Source: CAD feature listing. Evaluate the final solid. Frame: model axes, mm. Face numbers are marked on the shaded views. Coordinates: 2 decimals unless noted, no trailing zeros. Order: outer loops, then holes, each group sorted by start corner. A loop starts at its lowest first (then second) coordinate and runs counter-clockwise, first axis right, second up.
```python
from build123d import *

# Parameters (mm, degrees)
SKETCH1_W                = 9.525
SKETCH1_H                = 5.8
BOSS_EXTRUDE1_DEPTH      = 5.8
M3_CLEARANCE_HOLE1_D     = 3.2
M3_CLEARANCE_HOLE1_DEPTH = 12.7
M3_CLEARANCE_HOLE1_TIP   = 0.96137699
SKETCH5_R                = 0.5
CUT_EXTRUDE1_DEPTH       = 5.8


with BuildPart() as part:
    # Sketch1 → Boss-Extrude1 (new body)
    with BuildSketch(Plane.XY):
        with Locations((4.7625, 2.9)):
            Rectangle(SKETCH1_W, SKETCH1_H)
    extrude(amount=BOSS_EXTRUDE1_DEPTH)

    # M3 Clearance Hole1
    with Locations(Plane.XY.offset(5.8)):
        with Locations((6.35, 2.9)):
            Hole(M3_CLEARANCE_HOLE1_D / 2, depth=M3_CLEARANCE_HOLE1_DEPTH)
            with Locations((0, 0, -(M3_CLEARANCE_HOLE1_DEPTH + M3_CLEARANCE_HOLE1_TIP / 2))):  # 118° drill point
                Cone(0, M3_CLEARANCE_HOLE1_D / 2, M3_CLEARANCE_HOLE1_TIP, mode=Mode.SUBTRACT)

    # Sketch5 → Cut-Extrude1 (cut)
    with BuildSketch(Plane.XY.offset(5.8)):
        with Locations((2.38125, 4.2125)):
            Circle(SKETCH5_R)
    extrude(amount=-CUT_EXTRUDE1_DEPTH, mode=Mode.SUBTRACT)


solid = part.part
```
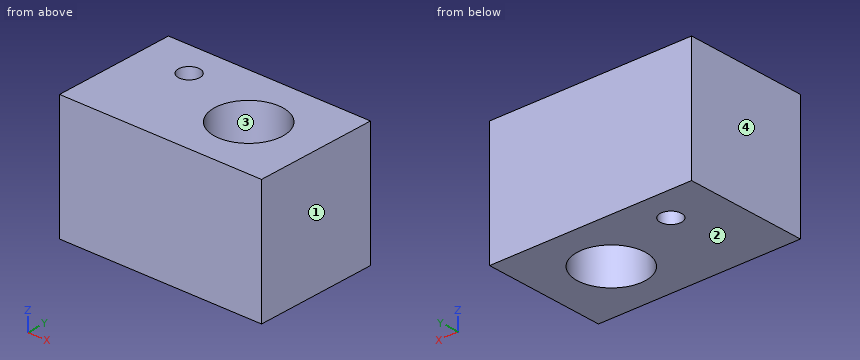
Q1. Material intervals for line 1 along Y through (x, z) = (6.35, 1.5); line 2 along X through (y, z) = (2.95, 2) (3 decimals); line 3 along X through (y, z) = (4.35, 2.05) (3 decimals), sorted ascending.
Solutions:
line 1: y = 0 to 1.3, 4.5 to 5.8
line 2: x = 0 to 4.751, 7.949 to 9.525
line 3: x = 0 to 1.901, 2.862 to 5.674, 7.026 to 9.525
Q2. Section query C-C on z = 1.8. Give the number of separate pieces and of enclosed holes in the cut face, plus the area to 3 significant figures.
Solutions:
separate pieces: 1
enclosed holes: 2
area: 46.4 mm2
Q3. Pull-direction query (X, two-part tool) for the marked faces 1, 2, 3 and 4; classes: pulls with the +X half, pulls with the -X half, needs draft (parallel to the pull), parting line crosses it, or undercut.
Solutions:
face 1: pulls with the +X half
face 2: needs draft
face 3: undercut
face 4: pulls with the -X half
Q4. Section query A-A on x = 6.35. Output: boundary loops of the cut face in (y, z), plus the area to 3 significant figures.
Solutions:
outline: (0, 0) - (1.3, 0) - (1.3, 5.8) - (0, 5.8) - close; (4.5, 0) - (5.8, 0) - (5.8, 5.8) - (4.5, 5.8) - close
area: 15.1 mm2
Q5. Section query B-B on y = 1.8. Output: boundary loops of the cut face in (x, z) (3 decimals).
Solutions:
outline: (0, 0) - (5.188, 0) - (5.188, 5.8) - (0, 5.8) - close; (7.512, 0) - (9.525, 0) - (9.525, 5.8) - (7.512, 5.8) - close
